For this review, take the finished solid that the model builds, in its own axes (mm). Give positions to 0.01 mm unless a question says otherwise; leave off trailing zeros. Write each loop counter-clockwise with the first axis right and the second up, starting at its lowest first coordinate (ties: lowest second). Pieces come first, ordered by that corner, then holes.
1) Wall thickness on line 1 along X through (y, z) = (-26.67, 0.95); line 2 along X through (y, z) = (-5, 0.7); line 3 along Y through (x, z) = (-9, 1.1): over which ranges is each line inside the solid? List them lowest first.
2) We need section A-A on y = -26.67. Give the boundary of the cut face in (x, z), and give its area (3 significant figures).
3) Draft analysis for pull direction Y (two halves, no side actions). For faces 1 (the face through (-1, 19, 0)), 2 (the face through (-34.753, -25.048, 0.751)), state which applies: pulls with the +Y half, pulls with the -Y half, needs draft (parallel to the pull), parting line crosses it, or undercut.
from build123d import *

# Parameters (mm, degrees)
SKETCH1_W                  = 84.328
SKETCH1_H                  = 165.1
SKETCH1_R                  = 1.8288
EXTRUDE1_DEPTH             = 1.524
SKETCH3_R                  = 0.635
LCD_HOLES_DEPTH            = 93.707216397
SKETCH4_R                  = 0.635
POT_HOLES_DEPTH            = 93.707216397
SKETCH5_R                  = 0.635
ARDUINO_HEADER_HOLES_DEPTH = 93.707216397
SKETCH6_W                  = 84.328
SKETCH6_H                  = 35.56
CUT_EXTRUDE1_DEPTH         = 93.707216397


with BuildPart() as part:
    # Sketch1 → Extrude1 (new body)
    with BuildSketch(Plane.XY):
        Rectangle(SKETCH1_W, SKETCH1_H)
        with Locations(Location((-38.989, 79.375, 0), (0, 0, 180))):
            Circle(SKETCH1_R, mode=Mode.SUBTRACT)
        with Locations(Location((38.989, 79.375, 0), (0, 0, 180))):
            Circle(SKETCH1_R, mode=Mode.SUBTRACT)
        with Locations(Location((-38.989, -79.375, 0), (0, 0, 180))):
            Circle(SKETCH1_R, mode=Mode.SUBTRACT)
        with Locations(Location((38.989, -79.375, 0), (0, 0, 180))):
            Circle(SKETCH1_R, mode=Mode.SUBTRACT)
        with Locations(Location((-33.909, -26.67, 0), (0, 0, 180))):
            Circle(SKETCH1_R, mode=Mode.SUBTRACT)
        with Locations(Location((34.671, -26.67, 0), (0, 0, 180))):
            Circle(SKETCH1_R, mode=Mode.SUBTRACT)
    extrude(amount=EXTRUDE1_DEPTH)

    # Sketch3 → LCD holes (cut, through all)
    with BuildSketch(Plane.XY.offset(1.524)):
        with Locations((-33.909, 69.85)):
            Circle(SKETCH3_R)
        with Locations((4.191, 69.85)):
            Circle(SKETCH3_R)
    extrude(amount=-LCD_HOLES_DEPTH, mode=Mode.SUBTRACT)

    # Sketch4 → Pot Holes (cut, through all)
    with BuildSketch(Plane.XY.offset(1.524)):
        with Locations((-33.909, 20.24)):
            Circle(SKETCH4_R)
        with Locations((-33.909, 10.24)):
            Circle(SKETCH4_R)
        with Locations((-8.509, 10.24)):
            Circle(SKETCH4_R)
        with Locations((-8.509, 20.24)):
            Circle(SKETCH4_R)
        with Locations((16.891, 10.24)):
            Circle(SKETCH4_R)
        with Locations((16.891, 20.24)):
            Circle(SKETCH4_R)
    extrude(amount=-POT_HOLES_DEPTH, mode=Mode.SUBTRACT)

    # Sketch5 → Arduino Header holes (cut, through all)
    with BuildSketch(Plane.XY.offset(1.524)):
        with Locations((-21.209, -5.16)):
            Circle(SKETCH5_R)
        with Locations((14.351, -5.16)):
            Circle(SKETCH5_R)
        with Locations((-21.209, -20.4)):
            Circle(SKETCH5_R)
        with Locations((14.351, -20.4)):
            Circle(SKETCH5_R)
    extrude(amount=-ARDUINO_HEADER_HOLES_DEPTH, mode=Mode.SUBTRACT)

    # Sketch6 → Cut-Extrude1 (cut, through all)
    with BuildSketch(Plane.XY.offset(1.524)):
        with Locations((0, -64.77)):
            Rectangle(SKETCH6_W, SKETCH6_H)
    extrude(amount=-CUT_EXTRUDE1_DEPTH, mode=Mode.SUBTRACT)


solid = part.part
Results list:
1. line 1: x = -42.16 to -35.74, -32.08 to 32.84, 36.5 to 42.16
1. line 2: x = -42.16 to -21.82, -20.59 to 13.74, 14.97 to 42.16
1. line 3: y = -46.99 to 9.84, 10.64 to 19.84, 20.64 to 82.55
2. outline: (-42.16, 0) - (-35.74, 0) - (-35.74, 1.52) - (-42.16, 1.52) - close; (-32.08, 0) - (32.84, 0) - (32.84, 1.52) - (-32.08, 1.52) - close; (36.5, 0) - (42.16, 0) - (42.16, 1.52) - (36.5, 1.52) - close
2. area: 117 mm2
3. face 1: needs draft
3. face 2: undercut
